Autodesk Fusion 360 part; units mm, degrees
sketch "Sketch1" plane through (0, 0, 0) normal (1, 0, 0) x (0, 0, -1)
  circle A0 centre (0, 0) radius 4
  line L0 (2, 2) -> (-2, 2)
  line L1 (-2, 2) -> (-2, -2)
  line L2 (-2, -2) -> (2, -2)
  line L3 (2, -2) -> (2, 2)
  line L4 (2, 2) -> (-2, -2) construction
  line L5 (-2, 2) -> (2, -2) construction
  dimension "d1" = 8
  dimension "d2" = 4
  dimension "d3" = 4
extrude "Extrude1" add sketch "Sketch1" along normal blind 2
sketch "Sketch2" plane through (2, 0, 0) normal (1, 0, 0) x (0, 0, -1)
  line L0 (2, 2) -> (2, -2)
  line L1 (2, -2) -> (-2, -2)
  line L2 (-2, -2) -> (-2, 2)
  line L3 (-2, 2) -> (2, 2)
  circle A0 centre (0, 0) radius 4
  circle A1 centre (0, 0) radius 7.5
  dimension "d6" = 15
extrude "Extrude2" add sketch "Sketch2" along normal blind 2 contours L0 L1 L2 L3 | A0 | A1
fillet "Fillet1" radius 1 1 edges at (2, -1.4465, 3.7293)
chamfer "Chamfer1" distance 0.5 angle 45 1 edges at (4, -2.7121, 6.9925)
sketch "Sketch3" plane through (4, 0, 0) normal (1, 0, 0) x (0, 0, -1)
  circle A0 centre (0, 0) radius 7
  line L0 (-2.5, 4.3301) -> (-2.5, -4.3301)
  line L1 (-2.5, -4.3301) -> (5, 0)
  line L2 (5, 0) -> (-2.5, 4.3301)
  dimension "d12" = 2.5
extrude "Extrude3" cut sketch "Sketch3" against normal blind 0.4 contours L0 L1 L2
Input: part model. Units: mm. Frame: model coordinates. A direction names the side the tool comes from. Give positions to 0.01 mm unless a question says otherwise; leave off trailing zeros. Order: outer loops, then holes, each group sorted by start corner. A loop starts at its lowest first (then second) coordinate and runs counter-clockwise, first axis right, second up.
1. Material intervals for L1, parallel to X at y = 4.75, z = 3; L2, parallel to Y at x = 0.8, z = -1.5; L3, parallel to Z at x = 1.8, y = -1.5, sorted ascending.
Derived:
L1: x = 2 to 4
L2: y = -3.71 to -2, 2 to 3.71
L3: z = -4.14 to -2, 2 to 4.14
2. Pin query (flat end, axial travel): pin 1 (1.5 mm diameter, centred on y = -0.5, z = -3.5, fed in from +X); pin 2 (2 mm diameter, centred on x = 1.5, z = -5, fed in from +Y); pin 3 (3 mm diameter, centred on y = 0, z = 0, fed in from -X); pin 4 (1 mm diameter, centred on x = 0.5, y = 0, fed in from +Z). Return the tip coordinate at first contact, or that it passes through.
Derived:
pin 1: stops at x = 4
pin 2: stops at y = 6.26
pin 3: stops at x = 2
pin 4: stops at z = 4
3. Section A-A on x = 1.75. Return the cut outline in (y, z), and give its area (3 significant figures).
Derived:
outline: circle Ø8.68 at (0, 0); hole (-2, -2) - (2, -2) - (2, 2) - (-2, 2) - close
area: 43.1 mm2
4. Section B-B on z = 0. Return the cut outline in (x, y).
Derived:
outline: (0, -4) - (1, -4) arc R1 cw to (2, -5) - (2, -7.5) - (3.5, -7.5) - (4, -7) - (4, -2.89) - (3.6, -2.89) - (3.6, 2.89) - (4, 2.89) - (4, 7) - (3.5, 7.5) - (2, 7.5) - (2, 5) arc R1 cw to (1, 4) - (0, 4) - (0, 2) - (2, 2) - (2, -2) - (0, -2) - close
5. Reachability of faces 1 (the flat face through (1, -2, 0)), 2 (the flat face through (3.803, 2.135, -1.302)), 3 (the flat face through (4, -3, -1)) from +Z, -Z, +X, -X, +Y, -Y: full face, straight path, thin tool, end or side. Return the list, or none.
Derived:
face 1: -X
face 2: +X
face 3: +Z, -Z, +X, +Y, -Y
6. Mould query, pull axis Z, two halves, no side actions, for faces 4 (the cylindrical face through (0.493, 3.905, 0.867)), 5 (the flat face through (0, 0, -3)), 6 (the flat face through (3.6, 0, 0)). Classes: released by +Z, released by -Z, zero draft, split by the parting line, or undercut.
Derived:
face 4: split by the parting line
face 5: zero draft
face 6: undercut
